Read the model definition and answer for the solid it produces. Units are mm, in the model's axes. Face numbers are marked on the shaded views. A direction names the side the tool comes from. Give positions to 0.01 mm unless a question says otherwise; leave off trailing zeros. Order: outer loops, then holes, each group sorted by start corner. A loop starts at its lowest first (then second) coordinate and runs counter-clockwise, first axis right, second up. Notation, with made-up numbers: (2.25, -0.75) - (44.25, -0.75) arc R23 cw to (44.25, 33.25) - close; hole circle Ø9 at (24, 83). An arc over 180 degrees is marked (long way). Write each question's results on one line, items separated by ' | '. Start each with the question number.
Q1. Find section A-A on y = 26.67. Give the vertices of the cut face in (x, z) (3 decimals), and give its area (3 significant figures).
Q2. Find the intervals of material crossed by line 1 along Y through (x, z) = (2.5, 3); line 2 along Y through (x, z) = (-21, 0) (3 decimals); line 3 along X through (y, z) = (40, 3.5), in increasing order. Write a range as from..to.
Q3. Flat-ended cylindrical pins translate along their axes: P1, Ø1, axis at x = 6.5, z = -7, coming from the +Y side; P2, Ø3, axis at y = 34.31, z = 0, coming from the +X side; P3, Ø7.5, axis at y = 59, z = 2, coming from the +X side. Find the tip coordinate at first contact, or state that the pin passes through.
Q4. A tool of negligible diameter and unlimited length cuts with its end or side. For the marked faces 1, 2 and 3, from which of +Z, -Z, +X, -X, +Y, -Y can it reach the whole face along a straight path? Write none if from no direction.
Q5. Find section C-C on z = -6.75. Give the vertices of the cut face in (x, y), and give its area (3 significant figures).
Q6. Find section B-B on z = 0. Give the vertices of the cut face in (x, y) (3 decimals).
Q7. For a pull along X with two mould halves and no side action, classify the marked faces 4, 5 and 6 as +X half, -X half, draft (parallel to the pull), parting line (faces both ways), or undercut.
Q8. Find section D-D on x = -4. Give the vertices of the cut face in (y, z).
from build123d import *

# Parameters (mm, degrees)
SKETCH1_W               = 50.8
SKETCH1_H               = 25.4
BOSS_EXTRUDE1_DEPTH     = 38.1
CUT_EXTRUDE1_DEPTH      = 53.363441445
CUT_EXTRUDE1_DEPTH_BACK = 53.363441445
SKETCH2_W               = 26.909263032
SKETCH2_H               = 12.7
CUT_EXTRUDE2_DEPTH      = 65.757547823
CUT_EXTRUDE2_DEPTH_BACK = 65.757547823
SKETCH3_R               = 1.905
SKETCH4_W               = 6.35
SKETCH4_H               = 25.4
BOSS_EXTRUDE2_DEPTH     = 38.1
CUT_EXTRUDE3_DEPTH      = 38.1


with BuildPart() as part:
    # Sketch1 → Boss-Extrude1 (new body)
    with BuildSketch(Plane(origin=(0, 0, 0), x_dir=(1, 0, 0), z_dir=(0, 1, 0))):
        Rectangle(SKETCH1_W, SKETCH1_H)
    extrude(amount=BOSS_EXTRUDE1_DEPTH)

    # Sketch2 → Cut-Extrude1 (cut, two sides: drawn at the far end of the back side and taken through both)
    with BuildSketch(Plane.XY.offset(12.7).offset(-CUT_EXTRUDE1_DEPTH_BACK)):
        with Locations((0, 26.67)):
            Rectangle(SKETCH2_W, SKETCH2_H)
    extrude(amount=CUT_EXTRUDE1_DEPTH + CUT_EXTRUDE1_DEPTH_BACK, mode=Mode.SUBTRACT)

    # Sketch3 → Cut-Extrude2 (cut, two sides: drawn at the far end of the back side and taken through both)
    with BuildSketch(Plane.ZY.offset(25.4).offset(-CUT_EXTRUDE2_DEPTH_BACK)):
        with Locations((0, 26.67)):
            Circle(SKETCH3_R)
    extrude(amount=CUT_EXTRUDE2_DEPTH + CUT_EXTRUDE2_DEPTH_BACK, mode=Mode.SUBTRACT)

    # Sketch4 → Boss-Extrude2 (add)
    with BuildSketch(Plane(origin=(0, 38.1, 0), x_dir=(1, 0, 0), z_dir=(0, 1, 0))):
        with Locations((-22.225, 0)):
            Rectangle(SKETCH4_W, SKETCH4_H)
    extrude(amount=BOSS_EXTRUDE2_DEPTH)

    # Sketch5 → Cut-Extrude3 (cut)
    with BuildSketch(Plane(origin=(25.4, 0, 0), x_dir=(0, 0, -1), z_dir=(1, 0, 0))):
        with BuildLine():
            Line((-1.254617423, 38.1), (1.254617423, 38.1))
            Line((1.254617423, 38.1), (1.254617423, 36.523684183))
            ThreePointArc((1.254617423, 36.523684183), (0, 31.773868069), (-1.254617423, 36.523684183))
            Line((-1.254617423, 36.523684183), (-1.254617423, 38.1))
        make_face()
    extrude(amount=-CUT_EXTRUDE3_DEPTH, mode=Mode.SUBTRACT)


solid = part.part
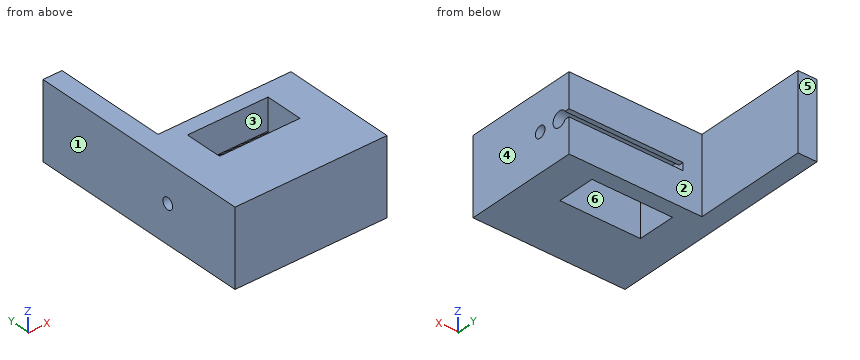
Working result:
1) outline: (-25.4, -12.7) - (-13.455, -12.7) - (-13.455, -1.905) - (-25.4, -1.905) - close; (-25.4, 1.905) - (-13.455, 1.905) - (-13.455, 12.7) - (-25.4, 12.7) - close; (13.455, -12.7) - (25.4, -12.7) - (25.4, -1.905) - (13.455, -1.905) - close; (13.455, 1.905) - (25.4, 1.905) - (25.4, 12.7) - (13.455, 12.7) - close | area: 516 mm²
2) line 1: 0..20.32, 33.02..38.1 | line 2: 0..24.765, 28.575..76.2 | line 3: -25.4..-19.05
3) P1: y = 38.1 | P2: x = -12.7 | P3: x = -19.05
4) face 1: +Z, -Z, -X, +Y, -Y | face 2: +Z, -Z, +X, +Y | face 3: +Z, -Z
5) outline: (-25.4, 0) - (25.4, 0) - (25.4, 38.1) - (-19.05, 38.1) - (-19.05, 76.2) - (-25.4, 76.2) - close; hole (-13.45, 20.32) - (13.45, 20.32) - (13.45, 33.02) - (-13.45, 33.02) - close | area: 1,840 mm²
6) outline: (-25.4, 0) - (25.4, 0) - (25.4, 24.765) - (13.455, 24.765) - (13.455, 20.32) - (-13.455, 20.32) - (-13.455, 24.765) - (-25.4, 24.765) - close; (-25.4, 28.575) - (-13.455, 28.575) - (-13.455, 33.02) - (-12.7, 33.02) - (-12.7, 38.1) - (-19.05, 38.1) - (-19.05, 76.2) - (-25.4, 76.2) - close; (13.455, 28.575) - (25.4, 28.575) - (25.4, 31.774) - (13.455, 31.774) - close
7) face 4: +X half | face 5: draft | face 6: undercut
8) outline: (0, -12.7) - (20.32, -12.7) - (20.32, 12.7) - (0, 12.7) - close; (33.02, -12.7) - (38.1, -12.7) - (38.1, -1.25) - (36.52, -1.25) arc R2.54 cw to (33.02, -2.19) - close; (33.02, 2.19) arc R2.54 cw to (36.52, 1.25) - (38.1, 1.25) - (38.1, 12.7) - (33.02, 12.7) - close
